Check sheet for the modelled part. Datum: model origin and axes. Units: mm. Give positions to 0.01 mm unless a question says otherwise; leave off trailing zeros. Loops run counter-clockwise (first coordinate to the right, second up) from the corner with the lowest first, then second, coordinate; pieces in that order, holes last. Notation, with made-up numbers: (25.5, 66.25) - (55.5, 66.25) arc R36 cw to (55.5, 100.25) - close; hole circle Ø8 at (13.5, 84.5). An arc over 180 degrees is marked (long way). Use one line per item in the form item = value.
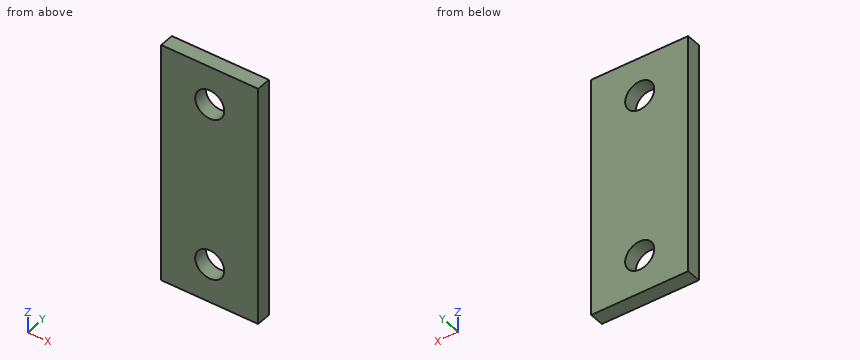
Autodesk Inventor part; units mm, degrees
ref_plane "YZ Plane" through (0, 0, 0) normal (1, 0, 0) x (0, 1, 0)
ref_plane "XZ Plane" through (0, 0, 0) normal (0, 1, 0) x (-1, 0, 0)
ref_plane "XY Plane" through (0, 0, 0) normal (0, 0, 1) x (1, 0, 0)
sketch "Skizze1" plane through (0, 0, 0) normal (0, 1, 0) x (-1, 0, 0)
  line L0 (0, 0) -> (-10, 0)
  line L1 (-10, 0) -> (-10, -25)
  line L2 (-10, -25) -> (0, -25)
  line L3 (0, -25) -> (0, 0)
  dimension "d0" = 10
  dimension "d1" = 25
extrude "Extrusion1" add sketch "Skizze1" along normal blind 1.5
sketch "Skizze2" plane through (0, 1.5, 0) normal (0, 1, 0) x (1, 0, 0)
  line L0 (0, 0) -> (10, 0)
  line L1 (10, 0) -> (10, 25)
  point P0 (5, 4)
  point P1 (5, 21)
  dimension "d4" = 17
  dimension "d6" = 4
  dimension "d7" = 5
  dimension "d8" = 5
hole "Bohrung1" at (5, 1.5, -4) at (5, 1.5, -21) direction (0, -1, 0) diameter 3 end through all
properties part number "montageplatte_rad_vorne"
Item 1: Thickness scan on L1, parallel to Z at x = 5, y = 0.6; L2, parallel to X at y = 0.7, z = -21; L3, parallel to Z at x = 3.75, y = 0.35. Record the ranges inside material, lowest first.
Answer block:
L1 = -25 to -22.5, -19.5 to -5.5, -2.5 to 0
L2 = 0 to 3.5, 6.5 to 10
L3 = -25 to -21.83, -20.17 to -4.83, -3.17 to 0
Item 2: Section check D-D on x = 6.25. Record the boundary of the cut face in (y, z), then the cut area to 3 significant figures.
Answer block:
outline = (0, -25) - (1.5, -25) - (1.5, -21.83) - (0, -21.83) - close; (0, -20.17) - (1.5, -20.17) - (1.5, -4.83) - (0, -4.83) - close; (0, -3.17) - (1.5, -3.17) - (1.5, 0) - (0, 0) - close
area = 32.5 mm2
Item 3: Section check A-A on z = -21. Record the boundary of the cut face in (x, y), then the cut area to 3 significant figures.
Answer block:
outline = (0, 0) - (3.5, 0) - (3.5, 1.5) - (0, 1.5) - close; (6.5, 0) - (10, 0) - (10, 1.5) - (6.5, 1.5) - close
area = 10.5 mm2
Item 4: Section check B-B on x = 5. Record the boundary of the cut face in (y, z).
Answer block:
outline = (0, -25) - (1.5, -25) - (1.5, -22.5) - (0, -22.5) - close; (0, -19.5) - (1.5, -19.5) - (1.5, -5.5) - (0, -5.5) - close; (0, -2.5) - (1.5, -2.5) - (1.5, 0) - (0, 0) - close
Item 5: Gauge pin test, flat end, axial feed: P1, Ø5, axis at x = 5, z = -4, coming from the +Y side. Record the tip position at first contact, or that the pin passes through.
Answer block:
P1 = 1.5
Item 6: Section check C-C on y = 1.2. Record the boundary of the cut face in (x, z).
Answer block:
outline = (0, -25) - (10, -25) - (10, 0) - (0, 0) - close; hole circle Ø3 at (5, -21); hole circle Ø3 at (5, -4)
